Geometry: final body of the model. Coordinates: model frame, mm. A direction names the side the tool comes from. Give positions to 0.01 mm unless a question says otherwise; leave off trailing zeros. Write each loop counter-clockwise with the first axis right and the second up, starting at its lowest first coordinate (ties: lowest second). Pieces come first, ordered by that corner, then holes. Notation, with made-up numbers: (71, 1) - (90, 1) arc R18 ccw to (90, 21) - close; hole circle Ø8 at (-32, -30.5). An arc over 180 degrees is marked (long way). Return JSON: item names as keys, results as strings.
Autodesk Fusion 360 part; units mm, degrees
sketch "Sketch1" plane through (0, 0, 0) normal (0, 1, 0) x (1, 0, 0)
  line L0 (0, 0) -> (40, 0)
  line L1 (40, 0) -> (40, -44)
  line L2 (40, -44) -> (0, -44)
  line L3 (0, -44) -> (0, 0)
  dimension "d1" = 40
  dimension "d2" = 44
extrude "Extrude1" add sketch "Sketch1" along normal blind 12.7
sketch "Sketch2" plane through (0, 12.7, 0) normal (0, 1, 0) x (-1, 0, 0)
  line L0 (0, 44) -> (-40, 44)
  line L1 (-40, 44) -> (-40, 0)
  line L2 (-40, 0) -> (0, 0)
  line L3 (0, 0) -> (0, 44)
  line L4 (0, 30.3) -> (-40, 30.3) construction
  point P0 (-20, 30.3)
  dimension "d38" = 30.3
hole "Hole8" at (20, 12.7, 30.3) direction (0, -1, 0) diameter 3.3 end through all
sketch "Sketch4" plane through (0, 0, 0) normal (0, 0, -1) x (-1, 0, 0)
  line L0 (-40, 0) -> (0, 0)
  line L1 (0, 0) -> (0, 12.7)
  line L2 (0, 12.7) -> (-40, 12.7)
  line L3 (-40, 12.7) -> (-40, 0)
  line L4 (-40, 7.7) -> (0, 7.7) construction
  line L5 (-20, 12.7) -> (-20, 0) construction
  point P0 (-35, 7.7)
  point P1 (-5, 7.7)
  point P2 (-20, 7.7)
  dimension "d39" = 5
  dimension "d40" = 15
  dimension "d41" = 15
hole "Hole9" at (35, 7.7, 0) direction (0, 0, 1) diameter 4.3 depth 10 tip angle 118
hole "Hole10" at (5, 7.7, 0) direction (0, 0, 1) diameter 4.3 depth 10 tip angle 118
hole "Hole11" at (20, 7.7, 0) direction (0, 0, 1) diameter 4.3 depth 10 tip angle 118
Q1. Mould query, pull axis Y, two halves, no side actions, for faces 3 (the flat face through (20, 0, 22)), 4 (the cylindrical face through (18.61, 6.26, 31.19)), 5 (the cylindrical face through (22.1, 7.23, 5.07)), 6 (the flat face through (20, 12.7, 22)). Classes: pulls with the +Y half, pulls with the -Y half, needs draft (parallel to the pull), parting line crosses it, or undercut.
Answer key:
{"face 3": "pulls with the -Y half", "face 4": "needs draft", "face 5": "undercut", "face 6": "pulls with the +Y half"}
Q2. Set-up query: faces 1 (the flat face through (20, 6, 44)), 2 (the cylindrical face through (32.87, 7.42, 5.07)). Return all of +Z, -Z, +X, -X, +Y, -Y with unobstructed straight access to the full face (end or side cutting, diameter ignored); none if empty.
Answer key:
{"face 1": "+Z, +X, -X, +Y, -Y", "face 2": "-Z"}
Q3. Section query A-A, the plane z = 30.3. Return the cut outline in (x, y), plus the area to 3 significant figures.
Answer key:
{"outline": "(0, 0) - (18.35, 0) - (18.35, 12.7) - (0, 12.7) - close; (21.65, 0) - (40, 0) - (40, 12.7) - (21.65, 12.7) - close", "area": "466 mm^2"}
Q4. Material intervals for probe 1 along X at (y, z) = (7.7, 7.5); probe 2 along X at (y, z) = (3, 30.5); probe 3 along Y at (x, z) = (35, 2), sorted ascending. Write a range as [from, to].
Answer key:
{"probe 1": "x = [0, 2.85], [7.15, 17.85], [22.15, 32.85], [37.15, 40]", "probe 2": "x = [0, 18.36], [21.64, 40]", "probe 3": "y = [0, 5.55], [9.85, 12.7]"}
Q5. Pin query (flat end, axial travel): P1, Ø10, axis at x = 20.5, z = 28.5, coming from the -Y side; P2, Ø3.5, axis at x = 5, y = 7.7, coming from the -Z side; P3, Ø3, axis at x = 20, z = 30.3, coming from the -Y side. Return the tip coordinate at first contact, or that it passes through.
Answer key:
{"P1": "stops at y = 0", "P2": "stops at z = 10.24", "P3": "passes through"}
